Build history of the part. All positions in model axes, mm. A direction names the side the tool comes from. Give positions to 0.01 mm unless a question says otherwise; leave off trailing zeros. Write each loop counter-clockwise with the first axis right and the second up, starting at its lowest first coordinate (ties: lowest second). Pieces come first, ordered by that corner, then holes. Notation, with made-up numbers: (26.25, 62) -> (70.25, 62) arc R23 cw to (70.25, 84) -> close; hole circle Ø2 at (71, -6). An arc over 180 degrees is marked (long way). Put each result on its own line as item: value.
from build123d import *

# Parameters (mm, degrees)
SKETCH1_R           = 2.286
BOSS_EXTRUDE1_DEPTH = 6.35
FILLET2_R           = 3.81
FILLET3_R           = 76.2


with BuildPart() as part:
    # Sketch1 → Boss-Extrude1 (new body)
    with BuildSketch(Plane(origin=(0, 0, 0), x_dir=(1, 0, 0), z_dir=(0, 1, 0))):
        with BuildLine():
            ThreePointArc((29.21, 30.48), (38.1, 39.37), (46.99, 30.48))
            Line((46.99, 30.48), (46.99, 18.8595))
            Line((46.99, 18.8595), (114.318469952, 18.8595))
            Line((114.318469952, 18.8595), (114.318469952, -3.4925))
            Line((114.318469952, -3.4925), (69.831530048, -3.4925))
            Line((69.831530048, -3.4925), (25.4, -19.05))
            Line((25.4, -19.05), (-25.4, -19.05))
            Line((-25.4, -19.05), (-69.831530048, -3.4925))
            Line((-69.831530048, -3.4925), (-114.281530048, -3.4925))
            Line((-114.281530048, -3.4925), (-114.281530048, 18.8595))
            Line((-114.281530048, 18.8595), (-46.99, 18.8595))
            Line((-46.99, 18.8595), (-46.99, 30.48))
            ThreePointArc((-46.99, 30.48), (-38.1, 39.37), (-29.21, 30.48))
            Line((-29.21, 30.48), (-29.21, 27.94))
            Line((-29.21, 27.94), (-9.321964372, 27.94))
            ThreePointArc((-9.321964372, 27.94), (0, 26.4795), (9.321964372, 27.94))
            Line((9.321964372, 27.94), (29.21, 27.94))
            Line((29.21, 27.94), (29.21, 30.48))
        make_face()
        with Locations(Location((101.581530048, 2.8575, 0), (0, 0, 270))):
            Circle(SKETCH1_R, mode=Mode.SUBTRACT)
        with Locations(Location((-101.581530048, 12.5095, 0), (0, 0, 270))):
            Circle(SKETCH1_R, mode=Mode.SUBTRACT)
        with Locations(Location((-101.581530048, 2.8575, 0), (0, 0, 270))):
            Circle(SKETCH1_R, mode=Mode.SUBTRACT)
        with Locations(Location((101.581530048, 12.5095, 0), (0, 0, 270))):
            Circle(SKETCH1_R, mode=Mode.SUBTRACT)
        with Locations(Location((-38.1, 30.48, 0), (0, 0, 270))):
            Circle(SKETCH1_R, mode=Mode.SUBTRACT)
        with Locations(Location((38.1, 30.48, 0), (0, 0, 270))):
            Circle(SKETCH1_R, mode=Mode.SUBTRACT)
        with BuildLine():
            Line((27.028870933, -4.475286106), (55.285884269, 5.809425657))
            ThreePointArc((55.285884269, 5.809425657), (56.087755755, 6.024286474), (56.914755201, 6.096639551))
            Line((56.914755201, 6.096639551), (61.58524071, 6.096639551))
            ThreePointArc((61.58524071, 6.096639551), (66.34774071, 10.859139551), (61.58524071, 15.621639551))
            Line((61.58524071, 15.621639551), (55.23524071, 15.621639551))
            ThreePointArc((55.23524071, 15.621639551), (54.408241264, 15.549286474), (53.606369777, 15.334425657))
            Line((53.606369777, 15.334425657), (25.349356441, 5.049713894))
            ThreePointArc((25.349356441, 5.049713894), (24.547484955, 4.834853076), (23.720485509, 4.7625))
            Line((23.720485509, 4.7625), (-23.720485509, 4.7625))
            ThreePointArc((-23.720485509, 4.7625), (-24.547484955, 4.834853076), (-25.349356441, 5.049713894))
            Line((-25.349356441, 5.049713894), (-53.606369777, 15.334425657))
            ThreePointArc((-53.606369777, 15.334425657), (-54.408241264, 15.549286474), (-55.23524071, 15.621639551))
            Line((-55.23524071, 15.621639551), (-61.58524071, 15.621639551))
            ThreePointArc((-61.58524071, 15.621639551), (-66.34774071, 10.859139551), (-61.58524071, 6.096639551))
            Line((-61.58524071, 6.096639551), (-56.914755201, 6.096639551))
            ThreePointArc((-56.914755201, 6.096639551), (-56.087755755, 6.024286474), (-55.285884269, 5.809425657))
            Line((-55.285884269, 5.809425657), (-27.028870933, -4.475286106))
            ThreePointArc((-27.028870933, -4.475286106), (-26.226999446, -4.690146924), (-25.4, -4.7625))
            Line((-25.4, -4.7625), (25.4, -4.7625))
            ThreePointArc((25.4, -4.7625), (26.226999446, -4.690146924), (27.028870933, -4.475286106))
        make_face(mode=Mode.SUBTRACT)
    extrude(amount=BOSS_EXTRUDE1_DEPTH)

    # Fillet2
    fillet2_edges = [part.edges().sort_by_distance(p)[0] for p in [
        (114.318469952, 3.175, -18.8595),
        (114.318469952, 3.175, 3.4925),
        (-114.281530048, 3.175, 3.4925),
        (-114.281530048, 3.175, -18.8595),
        (-9.321964372, 3.175, -27.94),
        (9.321964372, 3.175, -27.94),
    ]]
    fillet(fillet2_edges, radius=FILLET2_R)

    # Fillet3
    fillet3_edges = [part.edges().sort_by_distance(p)[0] for p in [
        (-46.99, 3.175, -18.8595),
        (-29.21, 3.175, -27.94),
        (29.21, 3.175, -27.94),
        (46.99, 3.175, -18.8595),
        (69.831530048, 3.175, 3.4925),
        (25.4, 3.175, 19.05),
        (-25.4, 3.175, 19.05),
        (-69.831530048, 3.175, 3.4925),
    ]]
    fillet(fillet3_edges, radius=FILLET3_R)


solid = part.part
1) Wall check: L1, parallel to Z at x = 1, y = 5; L2, parallel to Z at x = 44.5, y = 4.5; L3, parallel to Z at x = 95, y = 2.75. Give the ranges that are in metal, low to high.
Filled sheet:
L1: -26.5 to -4.76, 4.76 to 19.05
L2: -36.71 to -12.02, -1.88 to 12.36
L3: -18.86 to 3.49
2) Slice it at B-B (y = 4). Give the number of separate pieces and of enclosed holes in the cut face, plus the area to 3 significant figures.
Filled sheet:
separate pieces: 1
enclosed holes: 7
area: 6,980 mm2
3) Tool access for faces 5 (the flat face through (-96, 3, 3.492)), 6 (the flat face through (-59, 3, -6.097)), 7 (the cylindrical face through (-0.12, 3.13, -26.48)): list every direction of +Z, -Z, +X, -X, +Y, -Y with a clear straight run to the whole face (end or side of a thin tool).
Filled sheet:
face 5: +Z, -X, +Y, -Y
face 6: +Y, -Y
face 7: -Z, +Y, -Y
4) Pin check, flat tips, straight feed: pin 1 (3 mm diameter, centred on x = -11, y = 2.5, fed in from -Z); pin 2 (1 mm diameter, centred on x = -24, y = 5, fed in from -Z); pin 3 (2.5 mm diameter, centred on x = -38.1, z = -30.48, fed in from +Y); pin 4 (3.5 mm diameter, centred on x = -59.5, y = 4.5, fed in from -Z). Stop position of each tip, or through.
Filled sheet:
pin 1: z = -28.71
pin 2: z = -33.12
pin 3: through
pin 4: z = -27.77
5) Pull direction X, two halves, no side cores. Call faces 1 (the cylindrical face through (-103.813, 3.131, -13.005)), 2 (the cylindrical face through (38.644, 3.131, -39.353)), 3 (the cylindrical face through (-69.84, 3.22, 4.6)), 4 (the flat face through (2, 0, -11)): released by +X, released by -X, zero draft, split by the parting line, or undercut.
Filled sheet:
face 1: undercut
face 2: undercut
face 3: released by -X
face 4: zero draft
6) Slice it at A-A (z = -2.5). Write the cut outline in (x, y), plus the area to 3 significant figures.
Filled sheet:
outline: (-114.28, 0) -> (-103.84, 0) -> (-103.84, 6.35) -> (-114.28, 6.35) -> close; (-99.32, 0) -> (-46.19, 0) -> (-46.19, 6.35) -> (-99.32, 6.35) -> close; (46.19, 0) -> (99.32, 0) -> (99.32, 6.35) -> (46.19, 6.35) -> close; (103.84, 0) -> (114.32, 0) -> (114.32, 6.35) -> (103.84, 6.35) -> close
area: 808 mm2
